```python
from build123d import *

# Parameters (mm, degrees)
SKETCH1_R           = 0.5
BOSS_EXTRUDE1_DEPTH = 0.75
SKETCH2_R           = 0.19
CUT_EXTRUDE1_DEPTH  = 5.5
SKETCH3_R           = 0.375
CUT_EXTRUDE2_DEPTH  = 0.75


with BuildPart() as part:
    # Sketch1 → Boss-Extrude1 (new body, symmetric)
    with BuildSketch(Plane(origin=(0, 0, 0), x_dir=(1, 0, 0), z_dir=(0, 1, 0))):
        with BuildLine():
            Line((0, 1), (-4, 1))
            Line((-4, 1), (-4, 1.5))
            Line((-4, 1.5), (-3, 1.5))
            Line((-3, 1.5), (-0.00458684, 3))
            Line((-0.00458684, 3), (7.895751311, 3))
            ThreePointArc((7.895751311, 3), (8.3685457, 2.504929683), (8.75, 1.936491673))
            Line((8.75, 1.936491673), (8.75, 1.25))
            Line((8.75, 1.25), (7.75, 1.25))
            ThreePointArc((7.75, 1.25), (6.5, 0), (7.75, -1.25))
            Line((7.75, -1.25), (8.75, -1.25))
            Line((8.75, -1.25), (8.75, -1.936491673))
            ThreePointArc((8.75, -1.936491673), (8.3685457, -2.504929683), (7.895751311, -3))
            Line((7.895751311, -3), (-0.00458684, -3))
            Line((-0.00458684, -3), (-3, -1.5))
            Line((-3, -1.5), (-4, -1.5))
            Line((-4, -1.5), (-4, -1))
            Line((-4, -1), (0, -1))
            Line((0, -1), (0, 1))
        make_face()
        with Locations((5.25, 0)):
            Circle(SKETCH1_R, mode=Mode.SUBTRACT)
    extrude(amount=BOSS_EXTRUDE1_DEPTH, both=True)

    # Sketch2 → Cut-Extrude1 (cut, through all)
    with BuildSketch(Plane.XY.offset(1.5)):
        with Locations((-3.5, 0.4)):
            Circle(SKETCH2_R)
        with Locations((-3.5, -0.4)):
            Circle(SKETCH2_R)
    extrude(amount=-CUT_EXTRUDE1_DEPTH, mode=Mode.SUBTRACT)

    # Sketch3 → Cut-Extrude2 (cut)
    with BuildSketch(Plane.ZY):
        Circle(SKETCH3_R)
    extrude(amount=-CUT_EXTRUDE2_DEPTH, mode=Mode.SUBTRACT)


solid = part.part
```
CAD build for the part. Positions are in the model's coordinates, mm. A direction names the side the tool comes from. Coordinates: 2 decimals unless noted, no trailing zeros. Order: outer loops, then holes, each group sorted by start corner. A loop starts at its lowest first (then second) coordinate and runs counter-clockwise, first axis right, second up. Notation, with made-up numbers: M -21,-7.5 L 19,-7.5 A16 ccw 19,4.5 Z; hole C -4,38 d6. An arc over 180 degrees is marked long. Answer as CSV lines item,"result".
1) Cut at A-A (x = 5.25). List the corners of the cut face in (y, z), then the cut area to 3 significant figures.
Verdict:
outline,"M -0.75,-3 L 0.75,-3 L 0.75,-0.5 L -0.75,-0.5 Z; M -0.75,0.5 L 0.75,0.5 L 0.75,3 L -0.75,3 Z"
area,"7.50 mm2"
2) Cut at D-D (x = -3.5). List the corners of the cut face in (y, z), then the cut area to 3 significant figures.
Verdict:
outline,"M -0.75,-1.5 L -0.59,-1.5 L -0.59,-1 L -0.75,-1 Z; M -0.75,1 L -0.59,1 L -0.59,1.5 L -0.75,1.5 Z; M -0.21,-1.5 L 0.21,-1.5 L 0.21,-1 L -0.21,-1 Z; M -0.21,1 L 0.21,1 L 0.21,1.5 L -0.21,1.5 Z; M 0.59,-1.5 L 0.75,-1.5 L 0.75,-1 L 0.59,-1 Z; M 0.59,1 L 0.75,1 L 0.75,1.5 L 0.59,1.5 Z"
area,"0.740 mm2"
3) Mould opens along Z. For faces 6 (the flat face through (8, 0, 1.25)), 7 (the flat face through (4, 0, -3)), 8 (the flat face through (2, -0.75, 0)) say: released by +Z, released by -Z, zero draft, split by the parting line, or undercut.
Verdict:
face 6,"undercut"
face 7,"released by -Z"
face 8,"zero draft"
4) Flat gauge pins, fed straight in: P1, Ø0.5, axis at x = -3.5, y = 0.5, coming from the +Z side; P2, Ø0.5, axis at x = 8.5, y = -0.5, coming from the +Z side. Where does each tip first touch, or does it go through?
Verdict:
P1,"z = 1.5"
P2,"z = 2.65"
5) Drill centre lines: L1, parallel to Y at x = -3.5, z = -1.15; L2, parallel to Z at x = 7.75, y = 0.5; L3, parallel to X at y = 0.25, z = 0. Where is each one in solid material? Low to high. Write a range as from..to.
Verdict:
L1,"-0.75..-0.59, -0.21..0.21, 0.59..0.75"
L2,"-3..-1.25, 1.25..3"
L3,"0.75..4.75, 5.75..6.5"
6) 3-axis set-ups, long thin cutter, end or side, ignore diameter. For faces 1 (the flat face through (-3.5, 0, -1.5)), 2 (the flat face through (-2, 0, 1)), 3 (the flat face through (-3.5, 0, 1.5)), 4 (the flat face through (2, 0.75, 0)), 5 (the flat face through (8, 0, -1.25)): which of +Z, -Z, +X, -X, +Y, -Y reach the whole face in a straight line?
Verdict:
face 1,"-Z, -X, +Y, -Y"
face 2,"-X, +Y, -Y"
face 3,"+Z, -X, +Y, -Y"
face 4,"+Z, -Z, +X, -X, +Y"
face 5,"+X, +Y, -Y"
7) Cut at B-B (z = 0). List the corners of the cut face in (x, y) (3 decimals).
Verdict:
outline,"M 0,-0.75 L 4.75,-0.75 L 4.75,0.75 L 0,0.75 L 0,0.375 L 0.75,0.375 L 0.75,-0.375 L 0,-0.375 Z; M 5.75,-0.75 L 6.5,-0.75 L 6.5,0.75 L 5.75,0.75 Z"
